Geometry check sheet. Reference: the model listing, model coordinates, mm. A direction names the side the tool comes from. Round coordinates to 2 decimals unless told otherwise and drop trailing zeros. Order: outer loops, then holes, each group sorted by start corner. A loop starts at its lowest first (then second) coordinate and runs counter-clockwise, first axis right, second up. Notation, with made-up numbers: (0, -30.5) -> (12, -30.5) arc R21 ccw to (12, -8.5) -> close; hole circle Ø2 at (-14, 38). An arc over 180 degrees is marked (long way). Use a Markdown table: item, result. Add a question column.
Item 1: Material ranges on probe 1 along Y at (x, z) = (0.5, 9.5); probe 2 along Y at (x, z) = (0, 53), recorded low to high. Write a range as [from, to].
Item 2: Set-up check for faces 5 (the flat face through (-12.3, -19.3, 50.004)), 6 (the cylindrical face through (-9.45, -1.01, 40.49)), 7 (the flat face through (19, -2, 13)): record each of +Z, -Z, +X, -X, +Y, -Y from which the full face is reachable in a straight line by a thin tool's end or side.
Item 3: Mould release check, pull along Y, two halves, no side actions. Record for faces 1 (the cylindrical face through (-21.556, -6.788, 52.467)), 2 (the flat face through (-13, 13, 31)), 3 (the cylindrical face through (21.246, -8.809, 24.231)), 4 (the flat face through (2, 22, 55)): pulls with the +Y half, pulls with the -Y half, needs draft (parallel to the pull), parting line crosses it, or undercut.
Item 4: Sectioned sample at C-C, the plane y = 20. State how many separate pieces and enclosed holes the cut face has, and give its area (3 significant figures).
Item 5: Gauge pin test, flat ends, axial feed: pin 1 Ø14 at (x, y) = (3.5, -6.5) entering from +Z; pin 2 Ø3 at (x, z) = (-16.5, 31.5) entering from -Y (3 decimals); pin 3 Ø10.5 at (x, z) = (18, 12.5) entering from -Y; pin 4 Ø2 at (x, z) = (15.5, 43) entering from +Y. Record the tip position at first contact, or that the pin passes through.
Item 6: Sectioned sample at B-B, the plane z = 5.5. Record the cut outline in (x, y).
from build123d import *

# Parameters (mm, degrees)
F0_R           = 24
F1_DEPTH       = 50
F2_R           = 23
F3_DEPTH       = 50.001
F10_DEPTH      = 2
F13_DEPTH      = 2
F16_DEPTH      = 1
F16_DEPTH_BACK = 1
F19_DEPTH      = 2
F20_R          = 1


with BuildPart() as f1:
    # F0 (on Top) → F1 (new body)
    with BuildSketch(Plane.XY):
        Circle(F0_R)
    extrude(amount=F1_DEPTH)

    # F2 (on face) → F3 (cut, through all)
    with BuildSketch(Plane.XY.offset(50)):
        Circle(F2_R)
    extrude(amount=-F3_DEPTH, mode=Mode.SUBTRACT)

    # F4 (on Front) → F5 (revolve)
    with BuildSketch(Plane.XZ):
        Polygon((-22.6, 50.0044703981), (-23.5, 50.0044703981), (-23.5, 47.0044703981), (-21.6, 50), (-21.6, 55), (-22.6, 55), align=None)
    revolve(axis=Axis((0, 0, 50), (0, 0, 1)))

    # F9 (on Front) → F10 (join)
    with BuildSketch(Plane.XZ):
        Polygon((-8.5879870174, 40.5), (-23.5, 50), (-23.5, 31), align=None)
        Polygon((23.5, 6), (23.5, 20), (12.5122009602, 13), align=None)
    extrude(amount=F10_DEPTH)

    # F12 (on 3pt) → F13 (join)
    with BuildSketch(Plane(origin=(0, 0, 0), x_dir=(0.7071067812, -0.7071067812, 0), z_dir=(-0.7071067812, -0.7071067812, 0))):
        Polygon((-8.5879870174, 30.5), (-23.5, 40), (-23.5, 21), align=None)
    extrude(amount=F13_DEPTH)

    # F15 (on 3pt) → F16 (join, two sides)
    with BuildSketch(Plane.YZ) as f16_sk:
        Polygon((23.5, 11), (23.5, 30), (8.5879870174, 20.5), align=None)
    extrude(amount=-F16_DEPTH)
    extrude(f16_sk.sketch, amount=F16_DEPTH_BACK)

    # F18 (on 3pt) → F19 (join)
    with BuildSketch(Plane(origin=(0, 0, 0), x_dir=(0.7071067812, 0.7071067812, 0), z_dir=(0.7071067812, -0.7071067812, 0))):
        Polygon((23.5, 6), (23.5, 25), (8.5879870174, 15.5), align=None)
    extrude(amount=F19_DEPTH)

    # F20
    f20_edges = [f1.edges().sort_by_distance(p)[0] for p in [
        (-8.587987, -1, 40.5),
        (-6.779731, 5.365517, 30.5),
        (0, 8.587987, 20.5),
        (6.779731, 5.365517, 15.5),
        (12.512201, -1, 13),
    ]]
    fillet(f20_edges, radius=F20_R)


solid = f1.part
Found:
| question | item | result |
|---|---|---|
| 1 | probe 1 | y = [-23.99, -22.99], [22.99, 23.99] |
| 1 | probe 2 | y = [-22.6, -21.6], [21.6, 22.6] |
| 2 | face 5 | +Z |
| 2 | face 6 | none |
| 2 | face 7 | -Z |
| 3 | face 1 | parting line crosses it |
| 3 | face 2 | undercut |
| 3 | face 3 | undercut |
| 3 | face 4 | needs draft |
| 4 | separate pieces | 3 |
| 4 | enclosed holes | 0 |
| 4 | area | 250 mm2 |
| 5 | pin 1 | passes through |
| 5 | pin 2 | stops at y = -18.735 |
| 5 | pin 3 | stops at y = -20.33 |
| 5 | pin 4 | stops at y = 19.12 |
| 6 | outline | circle Ø48 at (0, 0); hole circle Ø46 at (0, 0) |
